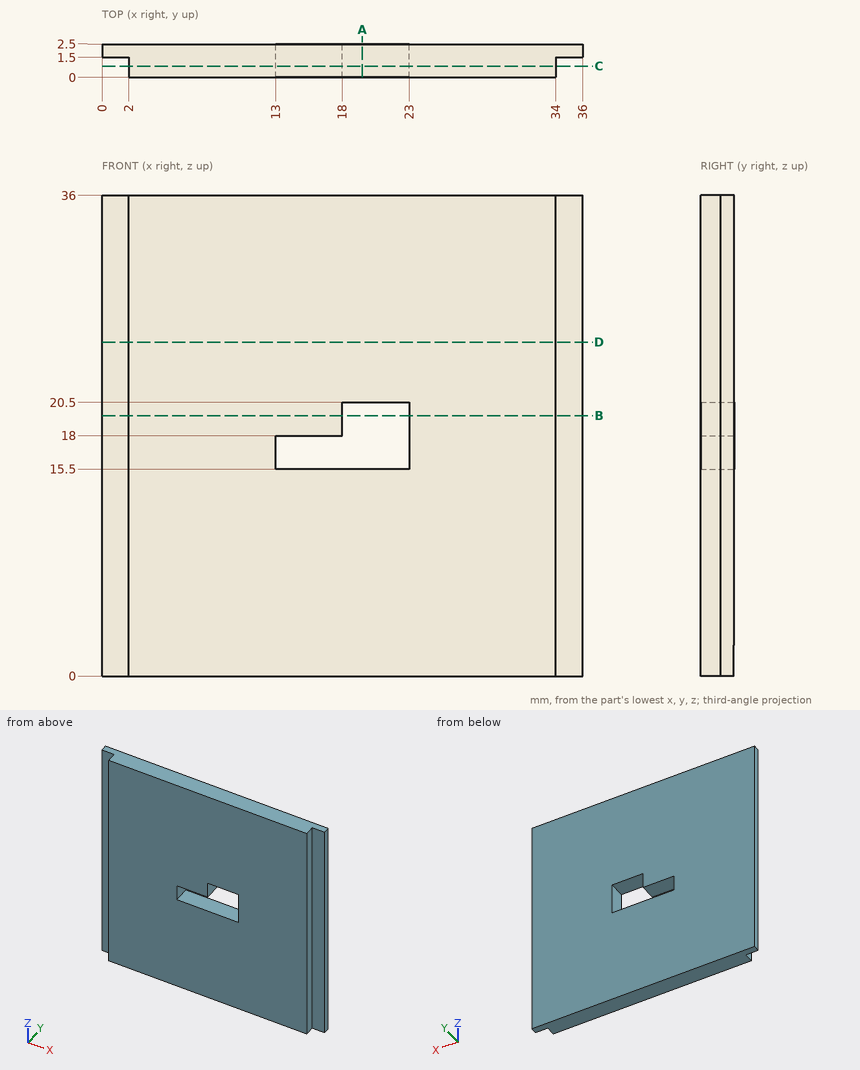
Job drawing, mm, ordinate dimensions from the low corner. One solid piece. Coordinates: 2 decimals unless noted, no trailing zeros. Loops run counter-clockwise (first coordinate to the right, second up) from the corner with the lowest first, then second, coordinate; pieces in that order, holes last. Notation, with made-up numbers: (36, 82.25) -> (69, 82.25) arc R29 ccw to (69, 111.25) -> close; hole circle Ø1 at (69.25, 51.5). An arc over 180 degrees is marked (long way). One line per item, written item: value.
1. Flat gauge pins, fed straight in: P1, Ø1.2, axis at y = 0.5, z = 16, coming from the +X side; P2, Ø1, axis at x = 35, z = 10, coming from the -Y side. Where does each tip first touch, or does it go through?
Answers:
P1: stops at x = 34
P2: stops at y = 1.5
2. Drill centre lines: line 1 (Z direction, x = 17.5, y = 0.55); line 2 (Z direction, x = 20, y = 0.9); line 3 (X direction, y = 1.2, z = 19.5). Where is each one in solid material? Low to high. Write a range as [from, to].
Answers:
line 1: z = [0, 15.5], [18, 36]
line 2: z = [0, 15.5], [20.5, 36]
line 3: x = [2, 18], [23, 34]
3. Slice it at C-C on y = 0.85. Write the cut outline in (x, z).
Answers:
outline: (2, 0) -> (34, 0) -> (34, 36) -> (2, 36) -> close; hole (13, 15.5) -> (23, 15.5) -> (23, 20.5) -> (18, 20.5) -> (18, 18) -> (13, 18) -> close
4. Slice it at B-B on z = 19.5. Write the cut outline in (x, y).
Answers:
outline: (0, 1.5) -> (2, 1.5) -> (2, 0) -> (18, 0) -> (18, 2.5) -> (0, 2.5) -> close; (23, 0) -> (34, 0) -> (34, 1.5) -> (36, 1.5) -> (36, 2.5) -> (23, 2.5) -> close
5. Slice it at A-A on x = 19.5. Write the cut outline in (y, z), and give its area (3 significant figures).
Answers:
outline: (0, 0) -> (2.5, 0) -> (2.5, 15.5) -> (0, 15.5) -> close; (0, 20.5) -> (2.5, 20.5) -> (2.5, 36) -> (0, 36) -> close
area: 77.5 mm^2
6. Slice it at D-D on z = 25. Write the cut outline in (x, y), and give its area (3 significant figures).
Answers:
outline: (0, 1.5) -> (2, 1.5) -> (2, 0) -> (34, 0) -> (34, 1.5) -> (36, 1.5) -> (36, 2.5) -> (0, 2.5) -> close
area: 84.0 mm^2
